from build123d import *

# Parameters (mm, degrees)
F0_R     = 12.5
F1_DEPTH = 12.4
F2_SIZE  = 1


with BuildPart() as f1:
    # F0 (on Top) → F1 (new body)
    with BuildSketch(Plane.XY):
        Circle(F0_R)
        with BuildLine():
            ThreePointArc((-4.1512046444, 1.3), (0, 4.35), (4.1512046444, 1.3))
            Line((4.1512046444, 1.3), (5, 1.3))
            Line((5, 1.3), (5, -1.3))
            Line((5, -1.3), (4.1512046444, -1.3))
            ThreePointArc((4.1512046444, -1.3), (0, -4.35), (-4.1512046444, -1.3))
            Line((-4.1512046444, -1.3), (-5, -1.3))
            Line((-5, -1.3), (-5, 1.3))
            Line((-5, 1.3), (-4.1512046444, 1.3))
        make_face(mode=Mode.SUBTRACT)
        with BuildLine():
            ThreePointArc((4.1512046444, -1.3), (4.3000139653, -0.657556004), (4.35, 0))
            ThreePointArc((4.35, 0), (4.3000139653, 0.657556004), (4.1512046444, 1.3))
            Line((4.1512046444, 1.3), (-4.1512046444, 1.3))
            ThreePointArc((-4.1512046444, 1.3), (-4.35, 0), (-4.1512046444, -1.3))
            Line((-4.1512046444, -1.3), (4.1512046444, -1.3))
        make_face()
        with BuildLine():
            ThreePointArc((4.1512046444, 1.3), (4.3000139653, 0.657556004), (4.35, 0))
            ThreePointArc((4.35, 0), (4.3000139653, -0.657556004), (4.1512046444, -1.3))
            Line((4.1512046444, -1.3), (5, -1.3))
            Line((5, -1.3), (5, 1.3))
            Line((5, 1.3), (4.1512046444, 1.3))
        make_face()
        with BuildLine():
            ThreePointArc((-4.1512046444, -1.3), (-4.35, 0), (-4.1512046444, 1.3))
            Line((-4.1512046444, 1.3), (-5, 1.3))
            Line((-5, 1.3), (-5, -1.3))
            Line((-5, -1.3), (-4.1512046444, -1.3))
        make_face()
    extrude(amount=F1_DEPTH)

    # F2
    f2_edges = [f1.edges().sort_by_distance(p)[0] for p in [
        (-12.5, 0, 12.4),
        (0, -4.35, 12.4),
        (0, -1.3, 12.4),
        (0, 1.3, 12.4),
        (0, 4.35, 12.4),
        (-12.5, 0, 0),
        (0, 1.3, 0),
        (0, 4.35, 0),
        (0, -1.3, 0),
        (0, -4.35, 0),
    ]]
    chamfer(f2_edges, length=F2_SIZE)


solid = f1.part
Read the model definition and answer for the solid it produces. Units are mm, in the model's axes. A direction names the side the tool comes from. Give positions to 0.01 mm unless a question says otherwise; leave off trailing zeros. Loops run counter-clockwise (first coordinate to the right, second up) from the corner with the lowest first, then second, coordinate; pieces in that order, holes last. Notation, with made-up numbers: M 9.5,84.25 L 57.5,84.25 A31 cw 57.5,110.25 Z; hole C -32,63 d9. An arc over 180 degrees is marked long. Write each question's results on one line, items separated by ' | '.
1. A tool of negligible diameter and unlimited length cuts with its end or side. For faces 4 (the face through (0, 1.3, 6)), 5 (the face through (0.1, -4.52, 11.57)), 6 (the face through (-0.1, 4.52, 0.83)), from which of +Z, -Z, +X, -X, +Y, -Y can it reach the whole face along a straight path? Write none if from no direction.
Values:
face 4: +Z, -Z | face 5: +Z | face 6: -Z
2. Straight lines are drawn through the part: line 1 (Y direction, x = 0.75, z = 8.75); line 2 (Y direction, x = 3, z = 9); line 3 (X direction, y = -2.75, z = 10). For each, find the intervals that lie inside material, in ascending order. Write a range as [from, to].
Values:
line 1: y = [-12.48, -4.28], [-1.3, 1.3], [4.28, 12.48] | line 2: y = [-12.13, -3.15], [-1.3, 1.3], [3.15, 12.13] | line 3: x = [-12.19, -3.37], [3.37, 12.19]
3. Given pin 1 (6 mm diameter, centred on x = 4.5, z = 6, fed in from +Y); pin 2 (1.5 mm diameter, centred on x = -6, z = 3, fed in from +Y); pin 3 (2.5 mm diameter, centred on x = 1.5, z = 4, fed in from +Y), each flat-ended and moving along its own axis, determine where each tip first touches the part or whether it passes through.
Values:
pin 1: stops at y = 12.41 | pin 2: stops at y = 11.34 | pin 3: stops at y = 12.5
4. The mould has two halves that part along Y. Classify faces 1 (the face through (0, 0, 0)), 2 (the face through (11.923, 3.755, 6.127)), 3 (the face through (0.1, 0.8, 0.5)): pulls with the +Y half, pulls with the -Y half, needs draft (parallel to the pull), parting line crosses it, or undercut.
Values:
face 1: needs draft | face 2: parting line crosses it | face 3: undercut
5. Section A-A on x = 0 is taken. Give the vertices of the cut face in (y, z).
Values:
outline: M -12.5,1 L -11.5,0 L -5.35,0 L -4.35,1 L -4.35,11.4 L -5.35,12.4 L -11.5,12.4 L -12.5,11.4 Z; M -1.3,1 L -0.3,0 L 0.3,0 L 1.3,1 L 1.3,11.4 L 0.3,12.4 L -0.3,12.4 L -1.3,11.4 Z; M 4.35,1 L 5.35,0 L 11.5,0 L 12.5,1 L 12.5,11.4 L 11.5,12.4 L 5.35,12.4 L 4.35,11.4 Z
6. Section B-B on z = 2 is taken. Give the vertices of the cut face in (x, y), plus the area to 3 significant figures.
Values:
outline: C 0,0 d25; hole M -4.15,-1.3 A4.35 ccw 4.15,-1.3 Z; hole M -4.15,1.3 L 4.15,1.3 A4.35 ccw Z | area: 454 mm^2
